```python
from build123d import *

# Parameters (mm, degrees)
SKETCH3_W                 = 75
SKETCH3_H                 = 254
BOSS_EXTRUDE2_DEPTH       = 35
SHELL2_T                  = -6
CUT_EXTRUDE1_DEPTH        = 2
CUT_EXTRUDE2_DEPTH        = 137.000919115
SKETCH6_W                 = 14
SKETCH6_H                 = 184
CUT_EXTRUDE3_DEPTH        = 152.58825812
FILLET1_R                 = 10
FILLET2_R                 = 5
SKETCH12_W                = 57.5
SKETCH12_H                = 8
BOSS_EXTRUDE4_DEPTH       = 35
FILLET5_R                 = 10
FILLET6_R                 = 15
M8X1_0_TAPPED_HOLE1_D     = 7
M8X1_0_TAPPED_HOLE1_DEPTH = 8
M8X1_0_TAPPED_HOLE1_TIP   = 2.103012167
SKETCH16_R                = 24
CUT_EXTRUDE4_DEPTH        = 91


with BuildPart() as part:
    # Sketch3 → Boss-Extrude2 (new body)
    with BuildSketch(Plane(origin=(0, 0, 0), x_dir=(0, 0, -1), z_dir=(1, 0, 0))):
        Rectangle(SKETCH3_W, SKETCH3_H)
    extrude(amount=BOSS_EXTRUDE2_DEPTH)

    # Shell2
    shell2_openings = [part.faces().sort_by_distance(p)[0] for p in [
        (35, 0, 0),
    ]]
    offset(amount=SHELL2_T, openings=shell2_openings, kind=Kind.INTERSECTION)

    # Sketch4 → Cut-Extrude1 (cut)
    with BuildSketch(Plane(origin=(6, 0, 0), x_dir=(0, 0, -1), z_dir=(1, 0, 0))):
        with BuildLine():
            Line((12.9, -5.439669108), (12.9, 5.439669108))
            ThreePointArc((12.9, 5.439669108), (0.363761531, 13.9952734), (-12.6, 6.102458521))
            Line((-12.6, 6.102458521), (-12.6, -6.102458521))
            ThreePointArc((-12.6, -6.102458521), (0.363761531, -13.9952734), (12.9, -5.439669108))
        make_face()
    extrude(amount=-CUT_EXTRUDE1_DEPTH, mode=Mode.SUBTRACT)

    # Sketch5 → Cut-Extrude2 (cut, through all)
    with BuildSketch(Plane(origin=(4, 0, 0), x_dir=(0, 0, -1), z_dir=(1, 0, 0))):
        with BuildLine():
            Line((9.9, -4.794788838), (9.9, 4.794788838))
            ThreePointArc((9.9, 4.794788838), (0, 11), (-9.9, 4.794788838))
            Line((-9.9, 4.794788838), (-9.9, -4.794788838))
            ThreePointArc((-9.9, -4.794788838), (0, -11), (9.9, -4.794788838))
        make_face()
    extrude(amount=-CUT_EXTRUDE2_DEPTH, mode=Mode.SUBTRACT)

    # Sketch6 → Cut-Extrude3 (cut, through all)
    with BuildSketch(Plane.XY.offset(37.5)):
        with Locations((17.5, 0)):
            Rectangle(SKETCH6_W, SKETCH6_H)
    extrude(amount=-CUT_EXTRUDE3_DEPTH, mode=Mode.SUBTRACT)

    # Fillet1
    fillet1_edges = [part.edges().sort_by_distance(p)[0] for p in [
        (17.5, -127, -37.5),
        (17.5, -127, 37.5),
        (17.5, 127, 37.5),
        (17.5, 127, -37.5),
    ]]
    fillet(fillet1_edges, radius=FILLET1_R)

    # Fillet2
    fillet2_edges = [part.edges().sort_by_distance(p)[0] for p in [
        (20.5, -121, -31.5),
        (20.5, 121, -31.5),
        (20.5, 121, 31.5),
        (20.5, -121, 31.5),
    ]]
    fillet(fillet2_edges, radius=FILLET2_R)

    # Sketch12 → Boss-Extrude4 (add)
    with BuildSketch(Plane(origin=(35, 0, 0), x_dir=(0, 0, -1), z_dir=(1, 0, 0))):
        with Locations((-66.25, -105)):
            Rectangle(SKETCH12_W, SKETCH12_H)
    extrude(amount=-BOSS_EXTRUDE4_DEPTH)

    # Fillet5
    # the kernel refuses this fillet: 10 mm, written as the material it adds along each edge
    with BuildSketch(Plane(origin=(35, -109, 37.5), x_dir=(0, -0.9999844906159053, -0.0055694279462415305), z_dir=(-1, 0, 0))) as fillet5_piece_1:
        with BuildLine():
            CenterArc((9.944708969, 9.955289483), FILLET5_R, 180.319106365, 84.260829523)
            Line((-0.055135937, 9.899595203), (-1.055120428, 9.894025775))
            Line((-1.055120428, 9.894025775), (-0.999984491, -0.005569428))
            Line((-0.999984491, -0.005569428), (0.005569428, -0.999984491))
            ThreePointArc((0.005569428, -0.999984491), (8.005445353, -0.955429067), (8.905682648, -0.995528948))
            Line((8.905682648, -0.995528948), (9.000139587, 0))
        make_face()
    extrude(amount=35)
    with BuildSketch(Plane(origin=(35, -101, 37.5), x_dir=(0, 1, 0), z_dir=(-1, 0, 0))) as fillet5_piece_2_section:
        with BuildLine():
            CenterArc((FILLET5_R, -FILLET5_R), FILLET5_R, 90, 90)
            Line((0, -FILLET5_R), (0, 0))
            Line((0, 0), (FILLET5_R, 0))
        make_face()
    fillet5_piece_2 = extrude(amount=35, mode=Mode.PRIVATE)
    fillet5_piece_2 = split(fillet5_piece_2, bisect_by=Plane(origin=(29.75, -92, 37.408860849), z_dir=(0, 1, 0)), keep=Keep.TOP, mode=Mode.PRIVATE)
    fillet5_piece_2 = split(fillet5_piece_2, bisect_by=Plane(origin=(24.5, -91.519267155, 37.408860849), z_dir=(1, 0, 0)), keep=Keep.TOP, mode=Mode.PRIVATE)
    add(fillet5_piece_2)
    with BuildSketch(Plane(origin=(35, -101, 37.5), x_dir=(0, 1, 0), z_dir=(-1, 0, 0))) as fillet5_piece_3_section:
        with BuildLine():
            CenterArc((FILLET5_R, -FILLET5_R), FILLET5_R, 90, 90)
            Line((0, -FILLET5_R), (0, 0))
            Line((0, 0), (FILLET5_R, 0))
        make_face()
    fillet5_piece_3 = extrude(amount=35, mode=Mode.PRIVATE)
    fillet5_piece_3 = split(fillet5_piece_3, bisect_by=Plane(origin=(29.75, -92, 39.784135406), z_dir=(0, -1, 0)), keep=Keep.TOP, mode=Mode.PRIVATE)
    fillet5_piece_3 = split(fillet5_piece_3, bisect_by=Plane(origin=(24.5, -98.797900168, 39.784135406), z_dir=(1, 0, 0)), keep=Keep.TOP, mode=Mode.PRIVATE)
    add(fillet5_piece_3)
    with BuildSketch(Plane(origin=(35, -101, 37.5), x_dir=(0, 1, 0), z_dir=(-1, 0, 0))) as fillet5_piece_4_section:
        with BuildLine():
            CenterArc((FILLET5_R, -FILLET5_R), FILLET5_R, 90, 90)
            Line((0, -FILLET5_R), (0, 0))
            Line((0, 0), (FILLET5_R, 0))
        make_face()
    fillet5_piece_4 = extrude(amount=35, mode=Mode.PRIVATE)
    fillet5_piece_4 = split(fillet5_piece_4, bisect_by=Plane(origin=(10.5, -98.797900168, 39.784135406), z_dir=(1, 0, 0)), keep=Keep.TOP, mode=Mode.PRIVATE)
    fillet5_piece_4 = split(fillet5_piece_4, bisect_by=Plane(origin=(17.5, -92, 39.784135406), z_dir=(0, -1, 0)), keep=Keep.TOP, mode=Mode.PRIVATE)
    fillet5_piece_4 = split(fillet5_piece_4, bisect_by=Plane(origin=(24.5, -98.797900168, 39.784135406), z_dir=(-1, 0, 0)), keep=Keep.TOP, mode=Mode.PRIVATE)
    add(fillet5_piece_4)
    with BuildSketch(Plane(origin=(35, -101, 37.5), x_dir=(0, 1, 0), z_dir=(-1, 0, 0))) as fillet5_piece_5_section:
        with BuildLine():
            CenterArc((FILLET5_R, -FILLET5_R), FILLET5_R, 90, 90)
            Line((0, -FILLET5_R), (0, 0))
            Line((0, 0), (FILLET5_R, 0))
        make_face()
    fillet5_piece_5 = extrude(amount=35, mode=Mode.PRIVATE)
    fillet5_piece_5 = split(fillet5_piece_5, bisect_by=Plane(origin=(10.5, -91.519267155, 37.408860849), z_dir=(-1, 0, 0)), keep=Keep.TOP, mode=Mode.PRIVATE)
    fillet5_piece_5 = split(fillet5_piece_5, bisect_by=Plane(origin=(5.25, -92, 37.408860849), z_dir=(0, 1, 0)), keep=Keep.TOP, mode=Mode.PRIVATE)
    add(fillet5_piece_5)
    with BuildSketch(Plane(origin=(35, -101, 37.5), x_dir=(0, 1, 0), z_dir=(-1, 0, 0))) as fillet5_piece_6_section:
        with BuildLine():
            CenterArc((FILLET5_R, -FILLET5_R), FILLET5_R, 90, 90)
            Line((0, -FILLET5_R), (0, 0))
            Line((0, 0), (FILLET5_R, 0))
        make_face()
    fillet5_piece_6 = extrude(amount=35, mode=Mode.PRIVATE)
    fillet5_piece_6 = split(fillet5_piece_6, bisect_by=Plane(origin=(10.5, -98.797900168, 39.784135406), z_dir=(-1, 0, 0)), keep=Keep.TOP, mode=Mode.PRIVATE)
    fillet5_piece_6 = split(fillet5_piece_6, bisect_by=Plane(origin=(5.25, -92, 39.784135406), z_dir=(0, -1, 0)), keep=Keep.TOP, mode=Mode.PRIVATE)
    add(fillet5_piece_6)

    # Fillet6
    fillet6_edges = [part.edges().sort_by_distance(p)[0] for p in [
        (35, -105, 95),
        (0, -105, 95),
    ]]
    fillet(fillet6_edges, radius=FILLET6_R)

    # M8x1.0 Tapped Hole1
    with Locations(Plane(origin=(17.5, -101, 62), x_dir=(0, 0, 1), z_dir=(0, 1, 0))):
        with Locations((0, 0)):
            Hole(M8X1_0_TAPPED_HOLE1_D / 2, depth=M8X1_0_TAPPED_HOLE1_DEPTH)
            with Locations((0, 0, -(M8X1_0_TAPPED_HOLE1_DEPTH + M8X1_0_TAPPED_HOLE1_TIP / 2))):  # 118° drill point
                Cone(0, M8X1_0_TAPPED_HOLE1_D / 2, M8X1_0_TAPPED_HOLE1_TIP, mode=Mode.SUBTRACT)

    # Sketch16 → Cut-Extrude4 (cut)
    with BuildSketch(Plane(origin=(0, -101, 0), x_dir=(1, 0, 0), z_dir=(0, 1, 0))):
        with Locations((17.5, -62)):
            Circle(SKETCH16_R)
    extrude(amount=CUT_EXTRUDE4_DEPTH, mode=Mode.SUBTRACT)


solid = part.part
```
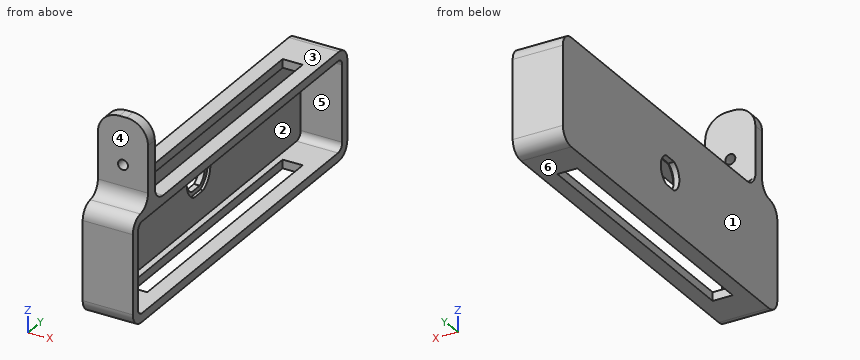
Read the model definition and answer for the solid it produces. Units are mm, in the model's axes. Face numbers are marked on the shaded views. A direction names the side the tool comes from. Round coordinates to 2 decimals unless told otherwise and drop trailing zeros. Write each loop counter-clockwise with the first axis right and the second up, starting at its lowest first coordinate (ties: lowest second). Pieces come first, ordered by that corner, then holes. Notation, with made-up numbers: (-0.75, 36.5) -> (45.25, 36.5) arc R19 ccw to (45.25, 41.5) -> close; hole circle Ø3 at (-28.5, -34). An arc over 180 degrees is marked (long way). Answer in a Markdown table with one row per item. Add a question column.
1) Find section B-B, the plane x = 17.5. State how many separate pieces and enclosed holes the cut face has, and give its area (3 significant figures).
2) Find section D-D, the plane y = 61. Determine the outline of the cut face in (x, z), and give its area (3 significant figures).
3) Given P1, Ø8.5, axis at x = 23.5, y = -57, coming from the +Z side; P2, Ø6.5, axis at y = 19, z = -36, coming from the -X side; P3, Ø6.5, axis at x = 20, z = 34, coming from the -Y side; P4, Ø13, axis at y = -5, z = 3, coming from the +X side, each flat-ended and moving along its own axis, determine where each tip first touches the part or whether it passes through.
4) Find section C-C, the plane z = 62. Determine the outline of the cut face in (x, y).
5) Consider line 1 (Z direction, x = 17.5, y = -106.75); line 2 (Z direction, x = 30.5, y = 66.5); line 3 (Y direction, x = 12, z = -21). Determine where each line is inside the solid, lowest interval first.
6) Determine the mould class of the marked faces 4, 5 and 6 for opening direction Z: pulls with the +Z half, pulls with the -Z half, needs draft (parallel to the pull), parting line crosses it, or undercut.
7) Which of the six approach directions +Z, -Z, +X, -X, +Y, -Y give full straight-line access (tool end or side, diameter ignored) to the marked faces 1, 2 and 3?
8) Find section A-A, the plane y = 0. Determine the outline of the cut face in (x, z).
Findings below:
| question | item | result |
|---|---|---|
| 1 | separate pieces | 3 |
| 1 | enclosed holes | 0 |
| 1 | area | 1,960 mm² |
| 2 | outline | (0, -37.5) -> (10.5, -37.5) -> (10.5, -31.5) -> (6, -31.5) -> (6, 31.5) -> (10.5, 31.5) -> (10.5, 37.5) -> (0, 37.5) -> close; (24.5, -37.5) -> (35, -37.5) -> (35, -31.5) -> (24.5, -31.5) -> close; (24.5, 31.5) -> (35, 31.5) -> (35, 37.5) -> (24.5, 37.5) -> close |
| 2 | area | 630 mm² |
| 3 | P1 | z = 37.5 |
| 3 | P2 | x = 0 |
| 3 | P3 | y = -126.46 |
| 3 | P4 | x = 4 |
| 4 | outline | (0, -109) -> (14, -109) -> (14, -101) -> (0, -101) -> close; (21, -109) -> (35, -109) -> (35, -101) -> (21, -101) -> close |
| 5 | line 1 | -37.5 to -31.5, 31.5 to 58.5, 65.5 to 95 |
| 5 | line 2 | -37.5 to -31.5, 31.5 to 37.5 |
| 5 | line 3 | -127 to -121, 121 to 127 |
| 6 | face 4 | needs draft |
| 6 | face 5 | undercut |
| 6 | face 6 | pulls with the -Z half |
| 7 | face 1 | +Z, -Z, -X, +Y, -Y |
| 7 | face 2 | +X |
| 7 | face 3 | +Z, +X, -X, +Y |
| 8 | outline | (0, -37.5) -> (10.5, -37.5) -> (10.5, -31.5) -> (6, -31.5) -> (6, -12.9) -> (4, -12.9) -> (4, -9.9) -> (0, -9.9) -> close; (0, 9.9) -> (4, 9.9) -> (4, 12.6) -> (6, 12.6) -> (6, 31.5) -> (10.5, 31.5) -> (10.5, 37.5) -> (0, 37.5) -> close; (24.5, -37.5) -> (35, -37.5) -> (35, -31.5) -> (24.5, -31.5) -> close; (24.5, 31.5) -> (35, 31.5) -> (35, 37.5) -> (24.5, 37.5) -> close |
